from build123d import *

# Parameters (mm, degrees)
SKETCH1_R               = 6.35
BOSS_EXTRUDE1_DEPTH     = 28.575
CUT_EXTRUDE1_DEPTH      = 28.575
CUT_EXTRUDE1_DEPTH_BACK = 28.575
SKETCH3_OUTSIDE_W       = 26.682
SKETCH3_OUTSIDE_H       = 26.682
SKETCH3_OUTSIDE_W_2     = 11.1125
SKETCH3_OUTSIDE_H_2     = 11.1125
CUT_EXTRUDE2_REACH      = 33.159


with BuildPart() as part:
    # Sketch1 → Boss-Extrude1 (new, symmetric)
    with BuildSketch(Plane.XY):
        Circle(SKETCH1_R)
    extrude(amount=BOSS_EXTRUDE1_DEPTH, both=True)

    # Sketch3 outside → Cut-Extrude1 (cut, two sides: drawn at the far end of the back side and taken through both)
    with BuildSketch(Plane.XY.offset(-CUT_EXTRUDE1_DEPTH_BACK)):
        Rectangle(SKETCH3_OUTSIDE_W, SKETCH3_OUTSIDE_H)
        Rectangle(SKETCH3_OUTSIDE_W_2, SKETCH3_OUTSIDE_H_2, mode=Mode.SUBTRACT)
    extrude(amount=CUT_EXTRUDE1_DEPTH + CUT_EXTRUDE1_DEPTH_BACK, mode=Mode.SUBTRACT)

    # Sketch4 → Cut-Extrude2 (cut, up to next)
    with BuildSketch(Plane.ZY.offset(5.55625), mode=Mode.PRIVATE) as cut_extrude2_sk1:
        with BuildLine():
            Line((-26.19375, 1.524), (-21.43125, 1.524))
            ThreePointArc((-21.43125, 1.524), (-19.90725, 0), (-21.43125, -1.524))
            Line((-21.43125, -1.524), (-26.19375, -1.524))
            ThreePointArc((-26.19375, -1.524), (-27.71775, 0), (-26.19375, 1.524))
        make_face()
    cut_extrude2_tool1 = extrude(cut_extrude2_sk1.sketch, amount=-CUT_EXTRUDE2_REACH, mode=Mode.PRIVATE) & part.part
    # Sketch4 → Cut-Extrude2 (cut, up to next)
    with BuildSketch(Plane.ZY.offset(5.55625), mode=Mode.PRIVATE) as cut_extrude2_sk2:
        with BuildLine():
            Line((26.19375, 1.524), (21.43125, 1.524))
            ThreePointArc((21.43125, 1.524), (19.90725, 0), (21.43125, -1.524))
            Line((21.43125, -1.524), (26.19375, -1.524))
            ThreePointArc((26.19375, -1.524), (27.71775, 0), (26.19375, 1.524))
        make_face()
    cut_extrude2_tool2 = extrude(cut_extrude2_sk2.sketch, amount=-CUT_EXTRUDE2_REACH, mode=Mode.PRIVATE) & part.part
    add(cut_extrude2_tool1.solids().sort_by_distance((-5.55625, 0, -23.8125))[0], mode=Mode.SUBTRACT)
    add(cut_extrude2_tool2.solids().sort_by_distance((-5.55625, 0, 23.8125))[0], mode=Mode.SUBTRACT)


solid = part.part
Read the model definition and answer for the solid it produces. Units are mm, in the model's axes. A direction names the side the tool comes from. Round coordinates to 2 decimals unless told otherwise and drop trailing zeros. Write each loop counter-clockwise with the first axis right and the second up, starting at its lowest first coordinate (ties: lowest second). Pieces come first, ordered by that corner, then holes.
1. Straight lines are drawn through the part: L1, parallel to Z at x = 1.5, y = -0.5 (3 decimals); L2, parallel to Z at x = 4, y = -1 (3 decimals); L3, parallel to Y at x = -1.5, z = 25.5. For each, find the intervals that lie inside material, in ascending order.
2. The part is cut by section B-B, the plane z = -14. Determine the outline of the cut face in (x, y).
3. Determine the mould class of faces 1 (the face through (-0.078, -0.034, 27.717)), 2 (the face through (-4.47, 4.51, 0.4)), 3 (the face through (0, -1.524, 24)), 4 (the face through (0, 0, -28.575)) for opening direction Y: pulls with the +Y half, pulls with the -Y half, needs draft (parallel to the pull), parting line crosses it, or undercut.
4. Which of the six approach directions +Z, -Z, +X, -X, +Y, -Y give full straight-line access (tool end or side, diameter ignored) to faces 5 (the face through (-0.078, 0.034, 19.908)), 6 (the face through (0, 0, 28.575))?
5. The part is cut by section A-A, the plane y = 0. Determine the outline of the cut face in (x, z) (3 decimals).
6. The part is cut by section D-D, the plane x = -3.75. Determine the outline of the cut face in (y, z) (3 decimals).
7. The part is cut by section C-C, the plane x = 1.25. Determine the outline of the cut face in (y, z) (3 decimals).
Values:
1. L1: z = -28.575 to -27.633, -19.992 to 19.992, 27.633 to 28.575
1. L2: z = -28.575 to -27.344, -20.281 to 20.281, 27.344 to 28.575
1. L3: y = -5.56 to -1.52, 1.52 to 5.56
2. outline: (-5.56, -3.07) arc R6.35 ccw to (-3.07, -5.56) - (3.07, -5.56) arc R6.35 ccw to (5.56, -3.07) - (5.56, 3.07) arc R6.35 ccw to (3.07, 5.56) - (-3.07, 5.56) arc R6.35 ccw to (-5.56, 3.07) - close
3. face 1: undercut
3. face 2: pulls with the +Y half
3. face 3: undercut
3. face 4: needs draft
4. face 5: +X, -X
4. face 6: +Z, +X, -X, +Y, -Y
5. outline: (-5.556, -28.575) - (5.556, -28.575) - (5.556, -27.718) - (-5.556, -27.718) - close; (-5.556, -19.907) - (5.556, -19.907) - (5.556, 19.907) - (-5.556, 19.907) - close; (-5.556, 27.718) - (5.556, 27.718) - (5.556, 28.575) - (-5.556, 28.575) - close
6. outline: (-5.124, -28.575) - (5.124, -28.575) - (5.124, 28.575) - (-5.124, 28.575) - close; hole (-1.524, -26.194) arc R1.524 ccw to (1.524, -26.194) - (1.524, -21.431) arc R1.524 ccw to (-1.524, -21.431) - close; hole (-1.524, 21.431) arc R1.524 ccw to (1.524, 21.431) - (1.524, 26.194) arc R1.524 ccw to (-1.524, 26.194) - close
7. outline: (-5.556, -28.575) - (5.556, -28.575) - (5.556, 28.575) - (-5.556, 28.575) - close; hole (-1.524, -26.194) arc R1.524 ccw to (1.524, -26.194) - (1.524, -21.431) arc R1.524 ccw to (-1.524, -21.431) - close; hole (-1.524, 21.431) arc R1.524 ccw to (1.524, 21.431) - (1.524, 26.194) arc R1.524 ccw to (-1.524, 26.194) - close
